Build history of the part. All positions in model axes, mm. Face numbers are marked on the shaded views. A direction names the side the tool comes from. Give positions to 0.01 mm unless a question says otherwise; leave off trailing zeros. Order: outer loops, then holes, each group sorted by start corner. A loop starts at its lowest first (then second) coordinate and runs counter-clockwise, first axis right, second up. Notation, with made-up numbers: M -1.75,4.5 L 11.25,4.5 A27 cw 11.25,25.5 Z; hole C -2,67 d7. An arc over 180 degrees is marked long. Answer as CSV lines item,"result".
Autodesk Inventor part; units mm, degrees
ref_plane "bracket_to_dummy_XY" through (0, 0, 0) normal (0, 1, 0) x (1, 0, 0)
ref_plane "bracket_to_dummy_YZ" through (0, 0, 0) normal (1, 0, 0) x (0, 0, -1)
ref_plane "bracket_to_dummy_ZX" through (0, 0, 0) normal (0, 0, -1) x (0, 1, 0)
sketch "Sketch_1" plane through (0, 0, 0) normal (1, 0, 0) x (0, 1, 0)
  line L0 (0, 80) -> (0, 0)
  line L1 (0, 0) -> (56.5685, 56.5685)
  line L2 (56.5685, 56.5685) -> (50.2046, 62.9325)
  line L3 (50.2046, 62.9325) -> (36.0624, 48.7904)
  line L4 (36.0624, 48.7904) -> (9, 60)
  line L5 (9, 60) -> (9, 80)
  line L6 (9, 80) -> (0, 80)
  arc A0 (6.8931, 25.3806) -> (5, 23.933) centre (6.5, 23.933) ccw
  line L7 (5, 23.933) -> (5, 15.6924)
  arc A1 (5, 15.6924) -> (7.5607, 14.6317) centre (6.5, 15.6924) ccw
  line L8 (7.5607, 14.6317) -> (13.3877, 20.4587)
  arc A2 (13.3877, 20.4587) -> (13.0726, 22.821) centre (12.327, 21.5194) ccw
  arc A3 (13.0726, 22.821) -> (6.8931, 25.3806) centre (0, 0) ccw
  circle A4 centre (12, 28.9706) radius 2.1
  arc A5 (7.074, 56.4682) -> (5, 55.0824) centre (6.5, 55.0824) ccw
  line L9 (5, 55.0824) -> (5, 32.7559)
  arc A6 (5, 32.7559) -> (7.5929, 31.7285) centre (6.5, 32.7559) ccw
  line L10 (7.5929, 31.7285) -> (8.2843, 32.4639)
  arc A7 (17.0976, 28.8133) -> (8.2843, 32.4639) centre (12, 28.9706) ccw
  line L11 (17.0976, 28.8133) -> (17.0665, 27.8044)
  arc A8 (17.0665, 27.8044) -> (19.6264, 26.6975) centre (18.5657, 27.7581) ccw
  line L12 (19.6264, 26.6975) -> (35.4136, 42.4847)
  arc A9 (35.4136, 42.4847) -> (34.927, 44.9311) centre (34.3529, 43.5453) ccw
  line L13 (34.927, 44.9311) -> (7.074, 56.4682)
extrude "Extrusion1" add sketch "Sketch_1" along normal mid plane 20
sketch "Sketch_2" plane through (-10, 50.2046, 62.9325) normal (0, -0.7071, 0.7071) x (1, 0, 0)
  circle A0 centre (10, -10) radius 3.5
extrude "Extrusion2" cut sketch "Sketch_2" against normal blind 9
sketch "Sketch_3" plane through (0, 0, 0) normal (0, 1, 0) x (-1, 0, 0)
  circle A0 centre (0, 70) radius 3.5
extrude "Extrusion3" cut sketch "Sketch_3" along normal blind 9
ref_plane "bracket_to_dummy_XY" through (0, 0, 0) normal (0, 1, 0) x (1, 0, 0)
ref_plane "bracket_to_dummy_YZ" through (0, 0, 0) normal (1, 0, 0) x (0, 0, -1)
ref_plane "bracket_to_dummy_ZX" through (0, 0, 0) normal (0, 0, -1) x (0, 1, 0)
ref_plane "1_to_bolt_XY" through (0, 9, 70) normal (0, 1, 0) x (1, 0, 0)
ref_plane "1_to_bolt_YZ" through (0, 9, 70) normal (1, 0, 0) x (0, 0, -1)
ref_plane "1_to_bolt_ZX" through (0, 9, 70) normal (0, 0, -1) x (0, 1, 0)
ref_plane "2_to_bolt_XY" through (0, 43.1335, 55.8614) normal (0, -0.7071, 0.7071) x (0, 0.7071, 0.7071)
ref_plane "2_to_bolt_YZ" through (0, 43.1335, 55.8614) normal (0, 0.7071, 0.7071) x (-1, 0, 0)
ref_plane "2_to_bolt_ZX" through (0, 43.1335, 55.8614) normal (-1, 0, 0) x (0, -0.7071, 0.7071)
ref_plane "3_to_bolt_XY" through (0, 9, 70) normal (0, 1, 0) x (0, 0, -1)
ref_plane "3_to_bolt_YZ" through (0, 9, 70) normal (0, 0, -1) x (-1, 0, 0)
ref_plane "3_to_bolt_ZX" through (0, 9, 70) normal (-1, 0, 0) x (0, 1, 0)
ref_plane "4_to_bolt_XY" through (30, 9, 70) normal (0, 1, 0) x (0, 0, -1)
ref_plane "4_to_bolt_YZ" through (30, 9, 70) normal (0, 0, -1) x (-1, 0, 0)
ref_plane "4_to_bolt_ZX" through (30, 9, 70) normal (-1, 0, 0) x (0, 1, 0)
ref_plane "5_to_bolt_XY" through (30, 43.1335, 55.8614) normal (0, -0.7071, 0.7071) x (0, 0.7071, 0.7071)
ref_plane "5_to_bolt_YZ" through (30, 43.1335, 55.8614) normal (0, 0.7071, 0.7071) x (-1, 0, 0)
ref_plane "5_to_bolt_ZX" through (30, 43.1335, 55.8614) normal (-1, 0, 0) x (0, -0.7071, 0.7071)
properties part number "HBL45TS6hbl45ts6"
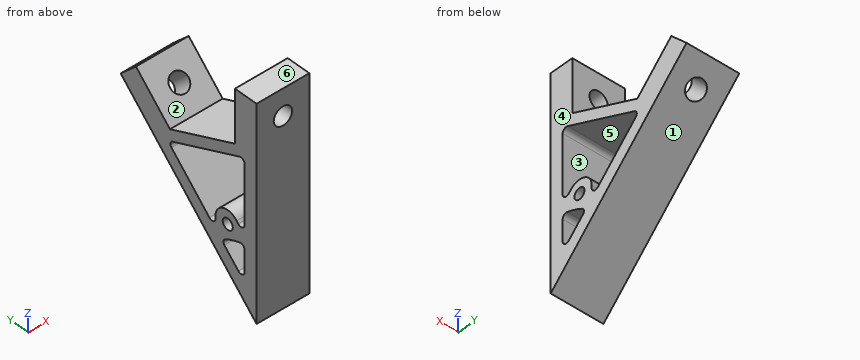
Item 1: Probe line 1 along Y through (x, z) = (2, 30.5); line 2 along Y through (x, z) = (0.25, 53); line 3 along Z through (x, y) = (4, 12). List the from-to ranges inside material, lowest first. Write a range as from..to.
Geometry says:
line 1,"y = 0..10.56, 13.44..16.87, 23.43..30.5"
line 2,"y = 0..5, 15.45..25.9, 40.27..41.06, 50.93..53"
line 3,"z = 12..19.07, 23.4..26.87, 31.07..34.07, 54.43..58.76"
Item 2: Drop flat-ended pins along their axis: pin 1 (12 mm diameter, centred on x = -3.5, y = 27.5, fed in from +Z); pin 2 (4 mm diameter, centred on y = 12, z = 28.97, fed in from +X); pin 3 (4 mm diameter, centred on x = 1, z = 20, fed in from +Y); pin 4 (1 mm diameter, centred on x = 5.5, y = 44.5, fed in from -Z). Give the stop position or say it passes through.
Geometry says:
pin 1,"stops at z = 54.82"
pin 2,"passes through"
pin 3,"stops at y = 22"
pin 4,"stops at z = 44"
Item 3: Band-saw the part on C-C (y = 15). Give the cut face in (x, z), and give its area (3 significant figures).
Geometry says:
outline,"M -10,15 L 10,15 L 10,33.09 L -10,33.09 Z; M -10,53.19 L 10,53.19 L 10,57.51 L -10,57.51 Z"
area,"448 mm2"
Item 4: Band-saw the part on A-A (x = -0.5). State how many separate pieces and enclosed holes the cut face has, and give its area (3 significant figures).
Geometry says:
separate pieces,"3"
enclosed holes,"3"
area,"1,020 mm2"
Item 5: 3-axis set-ups, long thin cutter, end or side, ignore diameter. For the marked faces 1, 2 and 3: which of +Z, -Z, +X, -X, +Y, -Y reach the whole face in a straight line?
Geometry says:
face 1,"-Z, +X, -X, +Y"
face 2,"+Z, +X, -X"
face 3,"+X, -X"
Item 6: Pull direction Z, two halves, no side cores. Call the marked faces 4, 5 and 6: released by +Z, released by -Z, zero draft, split by the parting line, or undercut.
Geometry says:
face 4,"zero draft"
face 5,"undercut"
face 6,"released by +Z"
Item 7: Band-saw the part on D-D (x = -5.75). Give the cut face in (y, z).
Geometry says:
outline,"M 0,0 L 56.57,56.57 L 50.2,62.93 L 36.06,48.79 L 9,60 L 9,80 L 0,80 Z; hole M 5,15.69 A1.5 ccw 7.56,14.63 L 13.39,20.46 A1.5 ccw 13.07,22.82 A26.3 ccw 6.89,25.38 A1.5 ccw 5,23.93 Z; hole M 5,32.76 A1.5 ccw 7.59,31.73 L 8.28,32.46 A5.1 cw 17.1,28.81 L 17.07,27.8 A1.5 ccw 19.63,26.7 L 35.41,42.48 A1.5 ccw 34.93,44.93 L 7.07,56.47 A1.5 ccw 5,55.08 Z; hole C 12,28.97 d4.2"
Item 8: Band-saw the part on B-B (z = 70). Give the cut face in (x, y), and give its area (3 significant figures).
Geometry says:
outline,"M -10,0 L -3.5,0 L -3.5,9 L -10,9 Z; M 3.5,0 L 10,0 L 10,9 L 3.5,9 Z"
area,"117 mm2"
